The figure shows three views and two pictorial views of one solid part (mm, origin at its lowest corner). Answer the questions. Round coordinates to 2 decimals unless told otherwise and drop trailing zeros. Order: outer loops, then holes, each group sorted by start corner. A loop starts at its lowest first (then second) coordinate and runs counter-clockwise, first axis right, second up. Notation, with made-up numbers: (0, 62) -> (57, 62) arc R8 cw to (57, 70) -> close; hole circle Ø4 at (86, -8). An arc over 180 degrees is marked (long way). Answer as a JSON object with one key per item and string values. Group by question number.
Item 1: Consider probe 1 along X at (y, z) = (1, 103); probe 2 along Z at (x, y) = (96.5, 8.75); probe 3 along X at (y, z) = (1.5, 107). Determine where each line is inside the solid, lowest interval first. Write a range as from..to.
Item 2: Section A-A, the plane x = 90 is taken. Count the separate pieces of the cut face and the enclosed holes in it, plus the area to 3 significant figures.
Item 3: Section B-B, the plane z = 90 is taken. Write down the section's boundary in (x, y), plus the area to 3 significant figures.
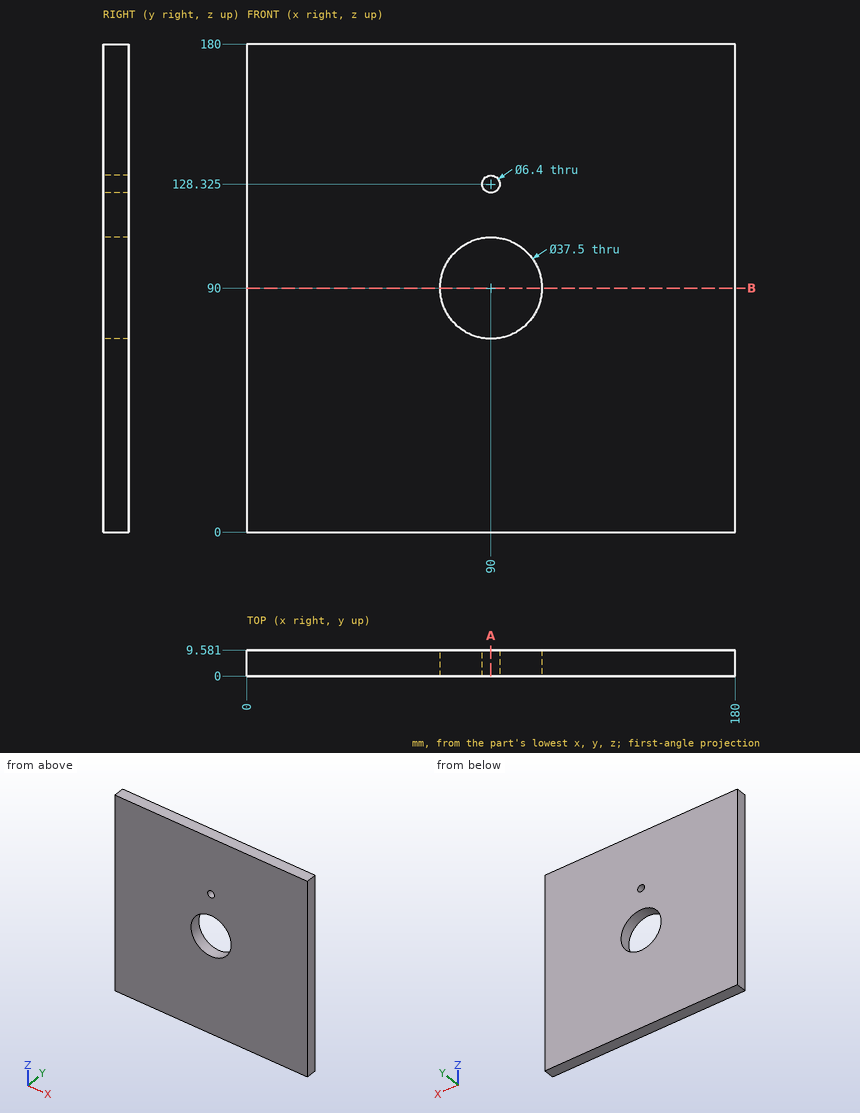
Values found:
{
 "1": {"probe 1": "0..76.49, 103.51..180", "probe 2": "0..72.41, 107.59..180", "probe 3": "0..82.09, 97.91..180"},
 "2": {"separate pieces": "3", "enclosed holes": "0", "area": "1,300 mm2"},
 "3": {"outline": "(0, 0) -> (71.25, 0) -> (71.25, 9.58) -> (0, 9.58) -> close; (108.75, 0) -> (180, 0) -> (180, 9.58) -> (108.75, 9.58) -> close", "area": "1,370 mm2"}
}
